```python
from build123d import *

# Parameters (mm, degrees)
F0_R        = 1
F1_DEPTH    = 15
F2_SIZE     = 3
F3_T1_DEPTH = 23.4240423609


# Not quite as in the source:
# - a fillet or chamfer that OpenCascade refuses, or shapes differently, is made with other operations: its cross-section is extruded or revolved along the edge and cut away or added


with BuildPart() as f1:
    # F0 (on Top) → F1 (new body)
    with BuildSketch(Plane.XY):
        with BuildLine():
            ThreePointArc((-4.5, 16.9115345253), (-10.6653645039, -13.8744369255), (17.5, 0))
            ThreePointArc((17.5, 0), (13.8744369255, 10.6653645039), (4.5, 16.9115345253))
            Line((4.5, 16.9115345253), (4.5, 0))
            ThreePointArc((4.5, 0), (0, -4.5), (-4.5, 0))
            Line((-4.5, 0), (-4.5, 16.9115345253))
        make_face()
        with Locations((0, -12)):
            Circle(F0_R, mode=Mode.SUBTRACT)
        with Locations((-10.3923048454, 6)):
            Circle(F0_R, mode=Mode.SUBTRACT)
        with Locations((10.3923048454, 6)):
            Circle(F0_R, mode=Mode.SUBTRACT)
    extrude(amount=F1_DEPTH)

    # F2
    f2_edges = [f1.edges().sort_by_distance(p)[0] for p in [
        (-10.665365, -13.874437, 15),
        (13.874437, 10.665365, 15),
    ]]
    chamfer(f2_edges, length=F2_SIZE)

    # F3: chamfer of 2 on 2 edges, made by hand

    # F3_s2 → F3_t1 (cut)
    with BuildSketch(Plane.XY.offset(-5.7120211805)):
        with BuildLine():
            Line((-6.685306539, 16.244612427), (-4.4335898165, 14.7321955637))
            Line((-4.4335898165, 14.7321955637), (-4.3935898165, 14.7321955637))
            ThreePointArc((-4.3935898165, 14.7321955637), (-4.46, 15.8218650445), (-4.46, 16.9115345253))
            Line((-4.46, 16.9115345253), (-4.5102857143, 16.9501894613))
            ThreePointArc((-4.5102857143, 16.9501894613), (-5.6067154961, 16.6197575598), (-6.700435445, 16.2816410133))
            Line((-6.700435445, 16.2816410133), (-6.685306539, 16.244612427))
        make_face()
        with BuildLine():
            Line((4.4335898165, 14.7321955637), (6.685306539, 16.244612427))
            Line((6.685306539, 16.244612427), (6.700435445, 16.2816410133))
            ThreePointArc((6.700435445, 16.2816410133), (5.6067154961, 16.6197575598), (4.5102857143, 16.9501894613))
            Line((4.5102857143, 16.9501894613), (4.46, 16.9115345253))
            ThreePointArc((4.46, 16.9115345253), (4.46, 15.8218650445), (4.3935898165, 14.7321955637))
            Line((4.3935898165, 14.7321955637), (4.4335898165, 14.7321955637))
        make_face()
    extrude(amount=F3_T1_DEPTH, mode=Mode.SUBTRACT)


solid = f1.part
```
Geometry: final body of the model. Coordinates: model frame, mm. A direction names the side the tool comes from. Give positions to 0.01 mm unless a question says otherwise; leave off trailing zeros. Loops run counter-clockwise (first coordinate to the right, second up) from the corner with the lowest first, then second, coordinate; pieces in that order, holes last. Notation, with made-up numbers: (6.25, 58) -> (49.25, 58) arc R15 ccw to (49.25, 82) -> close; hole circle Ø11 at (3, 42.5). An arc over 180 degrees is marked (long way). Return JSON: item names as keys, results as strings.
Item 1: Section D-D, the plane z = 12.5. Output: boundary loops of the cut face in (x, y).
Filled in:
{"outline": "(-6.12, 15.86) arc R17 ccw (long way) to (6.12, 15.86) -> (4.5, 14.78) -> (4.5, 0) arc R4.5 cw to (-4.5, 0) -> (-4.5, 14.78) -> close; hole circle Ø2 at (-10.39, 6); hole circle Ø2 at (0, -12); hole circle Ø2 at (10.39, 6)"}
Item 2: Section C-C, the plane y = 6. Count the separate pieces of the cut face and the enclosed holes in it, plus the area to 3 significant figures.
Filled in:
{"separate pieces": "4", "enclosed holes": "0", "area": "289 mm^2"}
Item 3: Line query: line 1 (Y direction, x = 0, z = 4.5); line 2 (X direction, y = 9, z = 8.25); line 3 (X direction, y = 4, z = 13.25). Output: solid intervals per line, ascending.
Filled in:
{"line 1": "-17.5 to -13, -11 to -4.5", "line 2": "-15.01 to -4.5, 4.5 to 15.01", "line 3": "-15.75 to -4.5, 4.5 to 15.75"}
Item 4: Access query for faces 3 (the flat face through (-5.574, 15.498, 6.928)), 4 (the flat face through (4, -4, 0)). Directions: +Z, -Z, +X, -X, +Y, -Y. A direction counts if a zero-diameter tool reaches every point of the face in a straight line with its end or side. Return the directions, or none.
Filled in:
{"face 3": "+Z, -Z, +Y", "face 4": "-Z, +X, -X, +Y, -Y"}
Item 5: Pin query (flat end, axial travel): P1, Ø3, axis at y = 4.5, z = 6.5, coming from the -X side; P2, Ø1.8, axis at x = 0, y = -12, coming from the -Z side; P3, Ø1, axis at x = -9.5, z = 10.5, coming from the -Y side; P4, Ø6, axis at x = 5.5, z = 12, coming from the -Y side. Return the tip coordinate at first contact, or that it passes through.
Filled in:
{"P1": "x = -17.24", "P2": "through", "P3": "y = -15.01", "P4": "y = -17.32"}
Item 6: Mould query, pull axis X, two halves, no side actions, for faces 1 (the flat face through (-3.4, -3.3, 15)), 2 (the cylindrical face through (-10.52, 6.99, 7.4)). Classes: released by +X, released by -X, zero draft, split by the parting line, or undercut.
Filled in:
{"face 1": "zero draft", "face 2": "undercut"}
Item 7: Section B-B, the plane z = 8.5. Output: boundary loops of the cut face in (x, y), plus the area to 3 significant figures.
Filled in:
{"outline": "(-6.62, 16.2) arc R17.5 ccw (long way) to (6.62, 16.2) -> (4.5, 14.78) -> (4.5, 0) arc R4.5 cw to (-4.5, 0) -> (-4.5, 14.78) -> close; hole circle Ø2 at (-10.39, 6); hole circle Ø2 at (0, -12); hole circle Ø2 at (10.39, 6)", "area": "761 mm^2"}
Item 8: Section A-A, the plane x = 0. Output: boundary loops of the cut face in (y, z).
Filled in:
{"outline": "(-17.5, 0) -> (-13, 0) -> (-13, 15) -> (-14.5, 15) -> (-17.5, 12) -> close; (-11, 0) -> (-4.5, 0) -> (-4.5, 15) -> (-11, 15) -> close"}
